Can you work these out from the model? Positions are in its coordinate system, mm. Coordinates: 2 decimals unless noted, no trailing zeros. Order: outer loops, then holes, each group sorted by start corner. A loop starts at its lowest first (then second) coordinate and runs counter-clockwise, first axis right, second up. Notation, with made-up numbers: (23.25, 26.5) -> (50.25, 26.5) arc R35 ccw to (50.25, 65.5) -> close; hole circle Ø1 at (-29, -34.5). An arc over 180 degrees is marked (long way). Return JSON: item names as keys, results as strings. Group by question number.
1) If we section it at B-B, the plane x = -58: State how many separate pieces and enclosed holes the cut face has, then the cut area to 3 significant figures.
2) If I drill on probe 1 along X at (y, z) = (-349, -8.5); probe 2 along Z at (x, y) = (-94.5, -464); probe 3 along X at (y, z) = (-803, -3), over which ranges is the centre line in solid material (lowest first)? Write a range as from..to.
3) For pin 1 (8 mm diameter, centred on x = 126.5, z = -30, fed in from -Y); pin 2 (15 mm diameter, centred on x = 38, y = -221.5, fed in from -Z); pin 3 (9 mm diameter, centred on x = -78.5, y = -847.5, fed in from +Z), each with a flat end and sliding along its axis, tell me the tip position at first contact or that it passes through.
4) If we section it at A-A, the plane y = -667: Please give me the cut outline in (x, z).
from build123d import *

# Parameters (mm, degrees)
F1_DEPTH = 1200
F3_DEPTH = 270


with BuildPart() as f1:
    # F0 (on Front) → F1 (new body)
    with BuildSketch(Plane.XZ):
        with BuildLine():
            Line((-314.166387, 0), (-334.166387, 0))
            ThreePointArc((-334.166387, 0), (-337.701921, -1.464466), (-339.166387, -5))
            Line((-339.166387, -5), (-339.166387, -40))
            Line((-339.166387, -40), (-309.166387, -40))
            Line((-309.166387, -40), (-309.166387, -5))
            ThreePointArc((-309.166387, -5), (-310.630854, -1.464466), (-314.166387, 0))
        make_face()
    extrude(amount=F1_DEPTH)

    # F2 (on face) → F3 (join)
    with BuildSketch(Plane.YZ.offset(-309.166387)):
        with BuildLine():
            Line((-1076.357331, -16), (-1106.357331, -16))
            ThreePointArc((-1106.357331, -16), (-1109.892865, -17.464466), (-1111.357331, -21))
            Line((-1111.357331, -21), (-1111.357331, -23))
            ThreePointArc((-1111.357331, -23), (-1109.892865, -26.535534), (-1106.357331, -28))
            Line((-1106.357331, -28), (-1076.357331, -28))
            ThreePointArc((-1076.357331, -28), (-1072.821797, -26.535534), (-1071.357331, -23))
            Line((-1071.357331, -23), (-1071.357331, -21))
            ThreePointArc((-1071.357331, -21), (-1072.821797, -17.464466), (-1076.357331, -16))
        make_face()
        with BuildLine():
            Line((-946.357331, -23), (-946.357331, -21))
            ThreePointArc((-946.357331, -21), (-947.821797, -17.464466), (-951.357331, -16))
            Line((-951.357331, -16), (-981.357331, -16))
            ThreePointArc((-981.357331, -16), (-984.892865, -17.464466), (-986.357331, -21))
            Line((-986.357331, -21), (-986.357331, -23))
            ThreePointArc((-986.357331, -23), (-984.892865, -26.535534), (-981.357331, -28))
            Line((-981.357331, -28), (-951.357331, -28))
            ThreePointArc((-951.357331, -28), (-947.821797, -26.535534), (-946.357331, -23))
        make_face()
        with BuildLine():
            Line((-821.357331, -23), (-821.357331, -21))
            ThreePointArc((-821.357331, -21), (-822.821797, -17.464466), (-826.357331, -16))
            Line((-826.357331, -16), (-856.357331, -16))
            ThreePointArc((-856.357331, -16), (-859.892865, -17.464466), (-861.357331, -21))
            Line((-861.357331, -21), (-861.357331, -23))
            ThreePointArc((-861.357331, -23), (-859.892865, -26.535534), (-856.357331, -28))
            Line((-856.357331, -28), (-826.357331, -28))
            ThreePointArc((-826.357331, -28), (-822.821797, -26.535534), (-821.357331, -23))
        make_face()
        with BuildLine():
            Line((-696.357331, -23), (-696.357331, -21))
            ThreePointArc((-696.357331, -21), (-697.821797, -17.464466), (-701.357331, -16))
            Line((-701.357331, -16), (-731.357331, -16))
            ThreePointArc((-731.357331, -16), (-734.892865, -17.464466), (-736.357331, -21))
            Line((-736.357331, -21), (-736.357331, -23))
            ThreePointArc((-736.357331, -23), (-734.892865, -26.535534), (-731.357331, -28))
            Line((-731.357331, -28), (-701.357331, -28))
            ThreePointArc((-701.357331, -28), (-697.821797, -26.535534), (-696.357331, -23))
        make_face()
        with BuildLine():
            Line((-571.357331, -23), (-571.357331, -21))
            ThreePointArc((-571.357331, -21), (-572.821797, -17.464466), (-576.357331, -16))
            Line((-576.357331, -16), (-606.357331, -16))
            ThreePointArc((-606.357331, -16), (-609.892865, -17.464466), (-611.357331, -21))
            Line((-611.357331, -21), (-611.357331, -23))
            ThreePointArc((-611.357331, -23), (-609.892865, -26.535534), (-606.357331, -28))
            Line((-606.357331, -28), (-576.357331, -28))
            ThreePointArc((-576.357331, -28), (-572.821797, -26.535534), (-571.357331, -23))
        make_face()
        with BuildLine():
            Line((-446.357331, -23), (-446.357331, -21))
            ThreePointArc((-446.357331, -21), (-447.821797, -17.464466), (-451.357331, -16))
            Line((-451.357331, -16), (-481.357331, -16))
            ThreePointArc((-481.357331, -16), (-484.892865, -17.464466), (-486.357331, -21))
            Line((-486.357331, -21), (-486.357331, -23))
            ThreePointArc((-486.357331, -23), (-484.892865, -26.535534), (-481.357331, -28))
            Line((-481.357331, -28), (-451.357331, -28))
            ThreePointArc((-451.357331, -28), (-447.821797, -26.535534), (-446.357331, -23))
        make_face()
        with BuildLine():
            Line((-321.357331, -23), (-321.357331, -21))
            ThreePointArc((-321.357331, -21), (-322.821797, -17.464466), (-326.357331, -16))
            Line((-326.357331, -16), (-356.357331, -16))
            ThreePointArc((-356.357331, -16), (-359.892865, -17.464466), (-361.357331, -21))
            Line((-361.357331, -21), (-361.357331, -23))
            ThreePointArc((-361.357331, -23), (-359.892865, -26.535534), (-356.357331, -28))
            Line((-356.357331, -28), (-326.357331, -28))
            ThreePointArc((-326.357331, -28), (-322.821797, -26.535534), (-321.357331, -23))
        make_face()
        with BuildLine():
            Line((-196.357331, -23), (-196.357331, -21))
            ThreePointArc((-196.357331, -21), (-197.821797, -17.464466), (-201.357331, -16))
            Line((-201.357331, -16), (-231.357331, -16))
            ThreePointArc((-231.357331, -16), (-234.892865, -17.464466), (-236.357331, -21))
            Line((-236.357331, -21), (-236.357331, -23))
            ThreePointArc((-236.357331, -23), (-234.892865, -26.535534), (-231.357331, -28))
            Line((-231.357331, -28), (-201.357331, -28))
            ThreePointArc((-201.357331, -28), (-197.821797, -26.535534), (-196.357331, -23))
        make_face()
        with BuildLine():
            Line((-71.357331, -23), (-71.357331, -21))
            ThreePointArc((-71.357331, -21), (-72.821797, -17.464466), (-76.357331, -16))
            Line((-76.357331, -16), (-106.357331, -16))
            ThreePointArc((-106.357331, -16), (-109.892865, -17.464466), (-111.357331, -21))
            Line((-111.357331, -21), (-111.357331, -23))
            ThreePointArc((-111.357331, -23), (-109.892865, -26.535534), (-106.357331, -28))
            Line((-106.357331, -28), (-76.357331, -28))
            ThreePointArc((-76.357331, -28), (-72.821797, -26.535534), (-71.357331, -23))
        make_face()
    extrude(amount=F3_DEPTH)

    # F4: F1 across face


with BuildPart() as f1_1:
    add(f1.part)
    add(f1.part.mirror(Plane(origin=(-39.166387, -841.357331, -22), x_dir=(0, 1, 0), z_dir=(1, 0, 0))))


solid = f1_1.part
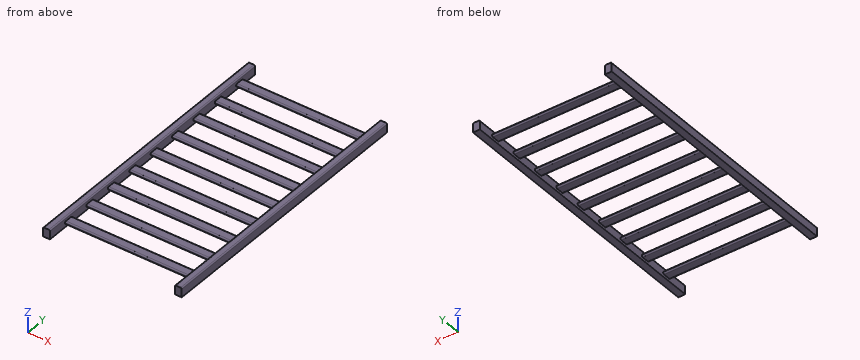
Result sheet:
{
 "1": {"separate pieces": "9", "enclosed holes": "0", "area": "4,130 mm2"},
 "2": {"probe 1": "x = -339.17..-309.17, 230.83..260.83", "probe 2": "z = -28..-16", "probe 3": "x = -338.75..-309.58, 231.25..260.42"},
 "3": {"pin 1": "stops at y = -1110.36", "pin 2": "stops at z = -28", "pin 3": "stops at z = -16"},
 "4": {"outline": "(-339.17, -40) -> (-309.17, -40) -> (-309.17, -5) arc R5 ccw to (-314.17, 0) -> (-334.17, 0) arc R5 ccw to (-339.17, -5) -> close; (230.83, -40) -> (260.83, -40) -> (260.83, -5) arc R5 ccw to (255.83, 0) -> (235.83, 0) arc R5 ccw to (230.83, -5) -> close"}
}
